Model file for the job. Use its own axes, mm. Face numbers are marked on the shaded views. A direction names the side the tool comes from. Coordinates: 2 decimals unless noted, no trailing zeros. Order: outer loops, then holes, each group sorted by start corner. A loop starts at its lowest first (then second) coordinate and runs counter-clockwise, first axis right, second up. Notation, with made-up numbers: (43, 77.25) -> (86, 77.25) arc R29 cw to (86, 110.25) -> close; hole circle Ø6 at (-29, 77.25). An arc over 180 degrees is marked (long way). Write item = value, one per line. Start each with the question number.
Q1. Mould opens along Y. For the marked faces 1, 2 and 3 say: +Y half, -Y half, draft (parallel to the pull), parting line (faces both ways), or undercut.
Q2. Flat gauge pins, fed straight in: pin 1 (1.5 mm diameter, centred on x = -17, y = 39, fed in from -Z); pin 2 (5 mm diameter, centred on x = 42.5, y = -46, fed in from +Z); pin 3 (8 mm diameter, centred on y = -16.5, z = 13.5, fed in from -X); pin 4 (3.5 mm diameter, centred on x = -54.5, y = 19, fed in from +Z). Where does each tip first touch, or does it go through?
Q3. Cut at C-C, the plane x = 8. List the corners of the cut face in (y, z), plus the area to 3 significant figures.
Q4. Cut at D-D, the plane z = 40.5. List the corners of the cut face in (x, y), plus the area to 3 significant figures.
Q5. Wall check: line 1 (X direction, y = -12, z = 23.5); line 2 (Y direction, x = -17, z = 18.5); line 3 (X direction, y = -54.5, z = 46). Give the ranges that are in metal, low to high. Write a range as from..to.
Q6. Cut at A-A, the plane z = 8.5. Give the number of separate pieces and of enclosed holes in the cut face, plus the area to 3 significant figures.
Q7. Cut at B-B, the plane z = 26. List the corners of the cut face in (x, y), plus the area to 3 significant figures.
Q8. 3-axis set-ups, long thin cutter, end or side, ignore diameter. For the marked faces 4, 5 and 6: which of +Z, -Z, +X, -X, +Y, -Y reach the whole face in a straight line?
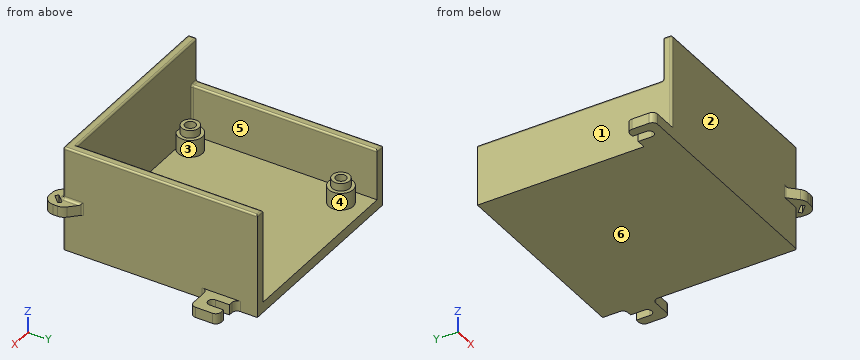
from build123d import *

# Parameters (mm, degrees)
SKETCH1_W            = 104.775
SKETCH1_H            = 106.3625
BOSS_EXTRUDE1_DEPTH  = 6
BOSS_EXTRUDE2_DEPTH  = 35
SKETCH3_R            = 5
SKETCH3_R_2          = 3.025
BOSS_EXTRUDE3_DEPTH  = 14.2875
SKETCH4_R            = 7
SKETCH4_R_2          = 3.025
BOSS_EXTRUDE4_DEPTH  = 9.8425
SKETCH6_W            = 15.875
SKETCH6_H            = 15.875
SKETCH6_W_2          = 15.88
SKETCH6_H_2          = 15.88
BOSS_EXTRUDE5_DEPTH  = 6
M5_CLEARANCE_HOLE2_D = 5.3
FILLET2_R            = 3
BOSS_EXTRUDE6_DEPTH  = 25
FILLET3_R            = 1
BOSS_EXTRUDE7_START  = 6
BOSS_EXTRUDE7_DEPTH  = 6
FILLET4_R            = 6
FILLET5_R            = 1.5
CUT_EXTRUDE1_DEPTH   = 113.041039013


with BuildPart() as part:
    # Sketch1 → Boss-Extrude1 (new body)
    with BuildSketch(Plane.XY):
        Rectangle(SKETCH1_W, SKETCH1_H)
    extrude(amount=BOSS_EXTRUDE1_DEPTH)

    # Sketch2 → Boss-Extrude2 (add)
    with BuildSketch(Plane.XY):
        Polygon((-57.3875, -53.18125), (-57.3875, -58.18125), (-52.3875, -58.18125), (57.3875, -58.18125), (57.3875, 53.18125), (52.3875, 53.18125), (52.3875, -53.18125), (-52.3875, -53.18125), (-52.3875, 53.18125), (-57.3875, 53.18125), align=None)
    extrude(amount=BOSS_EXTRUDE2_DEPTH)

    # Sketch3 → Boss-Extrude3 (add)
    # profile 1 of 4: a face of its own
    with BuildSketch(Plane.XY.offset(6)):
        with Locations((43.708, 39.35095)):
            Circle(SKETCH3_R)
        with Locations((43.708, 39.35095)):
            Circle(SKETCH3_R_2, mode=Mode.SUBTRACT)
    # profile 2 of 4: a face of its own
    with BuildSketch(Plane.XY.offset(6)):
        with Locations((-41.382, 39.35095)):
            Circle(SKETCH3_R)
        with Locations((-41.382, 39.35095)):
            Circle(SKETCH3_R_2, mode=Mode.SUBTRACT)
    # profile 3 of 4: a face of its own
    with BuildSketch(Plane.XY.offset(6)):
        with Locations((-41.382, -47.00905)):
            Circle(SKETCH3_R)
        with Locations((-41.382, -47.00905)):
            Circle(SKETCH3_R_2, mode=Mode.SUBTRACT)
    # profile 4 of 4: a face of its own
    with BuildSketch(Plane.XY.offset(6)):
        with Locations((43.708, -47.00905)):
            Circle(SKETCH3_R)
        with Locations((43.708, -47.00905)):
            Circle(SKETCH3_R_2, mode=Mode.SUBTRACT)
    extrude(amount=BOSS_EXTRUDE3_DEPTH)

    # Sketch4 → Boss-Extrude4 (add)
    # profile 1 of 4: a face of its own
    with BuildSketch(Plane.XY.offset(6)):
        with Locations((43.708, 39.35095)):
            Circle(SKETCH4_R)
        with Locations((43.708, 39.35095)):
            Circle(SKETCH4_R_2, mode=Mode.SUBTRACT)
    # profile 2 of 4: a face of its own
    with BuildSketch(Plane.XY.offset(6)):
        with Locations((-41.382, 39.35095)):
            Circle(SKETCH4_R)
        with Locations((-41.382, 39.35095)):
            Circle(SKETCH4_R_2, mode=Mode.SUBTRACT)
    # profile 3 of 4: a face of its own
    with BuildSketch(Plane.XY.offset(6)):
        with Locations((-41.382, -47.00905)):
            Circle(SKETCH4_R)
        with Locations((-41.382, -47.00905)):
            Circle(SKETCH4_R_2, mode=Mode.SUBTRACT)
    # profile 4 of 4: a face of its own
    with BuildSketch(Plane.XY.offset(6)):
        with Locations((43.708, -47.00905)):
            Circle(SKETCH4_R)
        with Locations((43.708, -47.00905)):
            Circle(SKETCH4_R_2, mode=Mode.SUBTRACT)
    extrude(amount=BOSS_EXTRUDE4_DEPTH)

    # Sketch6 → Boss-Extrude5 (add)
    with BuildSketch(Plane.XY):
        with Locations((65.325, 32.54375)):
            Rectangle(SKETCH6_W, SKETCH6_H)
        with Locations((-65.3275, -50.24125)):
            Rectangle(SKETCH6_W_2, SKETCH6_H_2)
    extrude(amount=BOSS_EXTRUDE5_DEPTH)

    # M5 Clearance Hole2 (through all)
    with Locations(Plane.XY.offset(6)):
        with Locations((65.325, 32.54375), (-65.3275, -50.24125)):
            Hole(M5_CLEARANCE_HOLE2_D / 2)

    # Fillet2
    fillet2_edges = [part.edges().sort_by_distance(p)[0] for p in [
        (-73.2675, -42.30125, 3),
        (-73.2675, -58.18125, 3),
        (73.2625, 24.60625, 3),
        (73.2625, 40.48125, 3),
        (57.3875, 40.48125, 3),
        (57.3875, 24.60625, 3),
    ]]
    fillet(fillet2_edges, radius=FILLET2_R)

    # Sketch9 → Boss-Extrude6 (add)
    with BuildSketch(Plane.XY.offset(35)):
        Polygon((52.3875, -53.18125), (-52.3875, -53.18125), (-57.3875, -53.18125), (-57.3875, -58.18125), (57.3875, -58.18125), (57.3875, 53.18125), (52.3875, 53.18125), align=None)
    extrude(amount=BOSS_EXTRUDE6_DEPTH)

    # Fillet3
    fillet3_edges = [part.edges().sort_by_distance(p)[0] for p in [
        (-52.3875, -53.18125, 20.5),
        (-57.3875, -58.18125, 33),
        (57.3875, -58.18125, 30),
        (-52.3875, 0, 35),
        (-54.8875, 53.18125, 35),
        (-57.3875, 0, 35),
        (-54.8875, -53.18125, 35),
        (-57.3875, -53.18125, 47.5),
        (-2.5, -53.18125, 60),
        (-57.3875, -55.68125, 60),
        (0, -58.18125, 60),
        (57.3875, -2.5, 60),
        (54.8875, 53.18125, 60),
        (52.3875, 0, 60),
    ]]
    fillet(fillet3_edges, radius=FILLET3_R)

    # Sketch10 → Boss-Extrude7 (add)
    with BuildSketch(Plane(origin=(0, 0, 30), x_dir=(-1, 0, 0), z_dir=(0, 0, -1)).offset(BOSS_EXTRUDE7_START)):
        with BuildLine():
            ThreePointArc((-56.3875, -58.18125), (-56.770183432, -58.105129533), (-57.094606781, -57.888356781))
            ThreePointArc((-57.094606781, -57.888356781), (-57.311379533, -57.563933432), (-57.3875, -57.18125))
            Line((-57.3875, -57.18125), (-57.3875, -47.18125))
            Line((-57.3875, -47.18125), (-64.544354249, -54.338104249))
            Line((-64.544354249, -54.338104249), (-64.544354249, -65.338104249))
            Line((-64.544354249, -65.338104249), (-53.544354249, -65.338104249))
            Line((-53.544354249, -65.338104249), (-46.3875, -58.18125))
            Line((-46.3875, -58.18125), (-56.3875, -58.18125))
        make_face()
        Polygon((-60.544354249, -56.838104249), (-56.044354249, -61.338104249), (-57.544354249, -62.838104249), (-62.044354249, -58.338104249), align=None, mode=Mode.SUBTRACT)
    extrude(amount=-BOSS_EXTRUDE7_DEPTH)

    # Fillet4
    fillet4_edges = [part.edges().sort_by_distance(p)[0] for p in [
        (64.544354249, -54.338104249, 27),
        (64.544354249, -65.338104249, 27),
        (53.544354249, -65.338104249, 27),
    ]]
    fillet(fillet4_edges, radius=FILLET4_R)

    # Fillet5
    fillet5_edges = [part.edges().sort_by_distance(p)[0] for p in [
        (57.3875, -52.18125, 30),
        (57.3875, -47.18125, 27),
        (51.3875, -58.18125, 30),
        (46.3875, -58.18125, 27),
        (57.094606781, -57.888356781, 30),
    ]]
    fillet(fillet5_edges, radius=FILLET5_R)

    # Sketch11 → Cut-Extrude1 (cut, through all)
    with BuildSketch(Plane.XY.offset(6)):
        with BuildLine():
            Line((-67.9775, -42.30125), (-67.9775, -50.24125))
            ThreePointArc((-67.9775, -50.24125), (-65.3275, -47.59125), (-62.6775, -50.24125))
            Line((-62.6775, -50.24125), (-62.6775, -42.30125))
            Line((-62.6775, -42.30125), (-67.9775, -42.30125))
        make_face()
        with BuildLine():
            Line((62.675, 40.48125), (62.675, 32.54375))
            ThreePointArc((62.675, 32.54375), (65.325, 35.19375), (67.975, 32.54375))
            Line((67.975, 32.54375), (67.975, 40.48125))
            Line((67.975, 40.48125), (62.675, 40.48125))
        make_face()
    extrude(amount=-CUT_EXTRUDE1_DEPTH, mode=Mode.SUBTRACT)


solid = part.part
Here are the results:
q1.face_1 = draft
q1.face_2 = -Y half
q1.face_3 = undercut
q2.pin_1 = 0
q2.pin_2 = 20.29
q2.pin_3 = -57.39
q2.pin_4 = 35
q3.outline = (-58.18, 0) -> (53.18, 0) -> (53.18, 6) -> (-53.18, 6) -> (-53.18, 59) arc R1 ccw to (-54.18, 60) -> (-57.18, 60) arc R1 ccw to (-58.18, 59) -> close
q3.area = 938 mm²
q4.outline = (-57.39, -57.18) arc R1 ccw to (-56.39, -58.18) -> (56.39, -58.18) arc R1 ccw to (57.39, -57.18) -> (57.39, 53.18) -> (52.39, 53.18) -> (52.39, -53.18) -> (-56.39, -53.18) arc R1 ccw to (-57.39, -54.18) -> close
q4.area = 1,110 mm²
q5.line_1 = -57.39..-52.39, 52.39..57.39
q5.line_2 = -58.18..-53.18
q5.line_3 = -57.39..57.39
q6.separate_pieces = 3
q6.enclosed_holes = 4
q6.area = 2,130 mm²
q7.outline = (-57.39, -57.18) arc R1 ccw to (-56.39, -58.18) -> (45.77, -58.18) arc R1.5 cw to (46.83, -58.62) -> (51.79, -63.58) arc R6 ccw to (56.03, -65.34) -> (58.54, -65.34) arc R6 ccw to (64.54, -59.34) -> (64.54, -56.82) arc R6 ccw to (62.79, -52.58) -> (57.83, -47.62) arc R1.5 cw to (57.39, -46.56) -> (57.39, 53.18) -> (52.39, 53.18) -> (52.39, -53.18) -> (-51.39, -53.18) arc R1 cw to (-52.39, -52.18) -> (-52.39, 53.18) -> (-57.39, 53.18) -> close; hole (56.04, -61.34) -> (57.54, -62.84) -> (62.04, -58.34) -> (60.54, -56.84) -> close
q7.area = 1,770 mm²
q8.face_4 = +Z
q8.face_5 = +Z, +Y
q8.face_6 = -Z, +X, -X, +Y, -Y
